```python
from build123d import *

# Parameters (mm, degrees)
F2_DEPTH      = 300
F3_W          = 8
F3_H          = 46
F4_DEPTH      = 5
F5_W          = 8
F5_H          = 46
F6_DEPTH      = 5
F7_W          = 50
F7_H          = 6
F8_DEPTH      = 5
F9_W          = 66
F9_H          = 45
F10_DEPTH     = 65.001
F11_R         = 2
F12_DEPTH     = 50.001
F13_T1_DEPTH  = 30
F13_T6_DEPTH  = 325
F13_T11_DEPTH = 325
F13_T16_DEPTH = 325
F13_T22_DEPTH = 325
F13_T27_DEPTH = 325
F13_T32_DEPTH = 325
F13_T37_DEPTH = 325
F13_T43_DEPTH = 325


# Not quite as in the source:
# - a fillet or chamfer that OpenCascade refuses, or shapes differently, is made with other operations: its cross-section is extruded or revolved along the edge and cut away or added


with BuildPart() as f2:
    # F1 (on face) → F2 (new body)
    with BuildSketch(Plane.XZ):
        Polygon((0, 0), (5, 0), (5, 45), (55, 45), (55, 0), (60, 0), (60, 50), (0, 50), align=None)
    extrude(amount=F2_DEPTH)

    # F3 (on face) → F4 (join)
    with BuildSketch(Plane.YZ.offset(60)):
        with Locations((-225, 25)):
            Rectangle(F3_W, F3_H)
        with Locations((-75, 25)):
            Rectangle(F3_W, F3_H)
    extrude(amount=F4_DEPTH)

    # F5 (on face) → F6 (join)
    with BuildSketch(Plane(origin=(0, 0, 0), x_dir=(0, -1, 0), z_dir=(-1, 0, 0))):
        with Locations((75, 25)):
            Rectangle(F5_W, F5_H)
        with Locations((225, 25)):
            Rectangle(F5_W, F5_H)
    extrude(amount=F6_DEPTH)

    # F7 (on face) → F8 (join)
    with BuildSketch(Plane(origin=(0, 0, 0), x_dir=(1, 0, 0), z_dir=(0, 0, -1))):
        with Locations((30, 74)):
            Rectangle(F7_W, F7_H)
        with Locations((30, 224)):
            Rectangle(F7_W, F7_H)
    extrude(amount=-F8_DEPTH)

    # F9 (on face) → F10 (cut, through all)
    with BuildSketch(Plane(origin=(0, 0, 0), x_dir=(0, -1, 0), z_dir=(-1, 0, 0))):
        Polygon((221, 45), (79, 45), (79, 2), (79, 0), (221, 0), (221, 2), align=None)
        with Locations((33, 22.5)):
            Rectangle(F9_W, F9_H)
        with Locations((267, 22.5)):
            Rectangle(F9_W, F9_H)
    extrude(amount=-F10_DEPTH, mode=Mode.SUBTRACT)

    # F11 (on Top) → F12 (cut, through all)
    with BuildSketch(Plane.XY):
        with Locations((-2.5, -75)):
            Circle(F11_R)
        with Locations((62.5, -75)):
            Circle(F11_R)
        with Locations((-2.5, -225)):
            Circle(F11_R)
        with Locations((62.5, -225)):
            Circle(F11_R)
    extrude(amount=F12_DEPTH, mode=Mode.SUBTRACT)

    # F13: fillet of radius 5 on 6 edges, made by hand

    # F13_s2 → F13_t1 (cut)
    with BuildSketch(Plane.XY.offset(32.5)):
        with BuildLine():
            ThreePointArc((0, -295), (1.4644660941, -298.5355339059), (5, -300))
            Line((5, -300), (0, -300))
            Line((0, -300), (0, -295))
        make_face()
        with BuildLine():
            ThreePointArc((60, -295), (58.5355339059, -298.5355339059), (55, -300))
            Line((55, -300), (60, -300))
            Line((60, -300), (60, -295))
        make_face()
        with BuildLine():
            ThreePointArc((60, -5), (58.5355339059, -1.4644660941), (55, 0))
            Line((55, 0), (60, 0))
            Line((60, 0), (60, -5))
        make_face()
        with BuildLine():
            ThreePointArc((0, -5), (1.4644660941, -1.4644660941), (5, 0))
            Line((5, 0), (0, 0))
            Line((0, 0), (0, -5))
        make_face()
    extrude(amount=F13_T1_DEPTH, mode=Mode.SUBTRACT)


with BuildPart() as f13_tool4:
    # F13_s5 → F13_t6 (new body)
    with BuildSketch(Plane.XZ.offset(-12.5)):
        with BuildLine():
            ThreePointArc((0, 45), (1.4644660941, 48.5355339059), (5, 50))
            Line((5, 50), (0, 50))
            Line((0, 50), (0, 45))
        make_face()
    extrude(amount=F13_T6_DEPTH)

    split(bisect_by=Plane.XZ.offset(71), keep=Keep.BOTTOM)


with BuildPart() as f2_1:
    add(f2.part)

    # F13_t3: cut F13_tool4
    add(f13_tool4.part, mode=Mode.SUBTRACT)


with BuildPart() as f13_tool9:
    # F13_s10 → F13_t11 (new body)
    with BuildSketch(Plane.XZ.offset(-12.5)):
        with BuildLine():
            ThreePointArc((0, 45), (1.4644660941, 48.5355339059), (5, 50))
            Line((5, 50), (0, 50))
            Line((0, 50), (0, 45))
        make_face()
    extrude(amount=F13_T11_DEPTH)

    split(bisect_by=Plane.XY.offset(48), keep=Keep.TOP)


with BuildPart() as f2_2:
    add(f2_1.part)

    # F13_t8: cut F13_tool9
    add(f13_tool9.part, mode=Mode.SUBTRACT)


with BuildPart() as f13_tool14:
    # F13_s15 → F13_t16 (new body)
    with BuildSketch(Plane.XZ.offset(-12.5)):
        with BuildLine():
            ThreePointArc((0, 45), (1.4644660941, 48.5355339059), (5, 50))
            Line((5, 50), (0, 50))
            Line((0, 50), (0, 45))
        make_face()
    extrude(amount=F13_T16_DEPTH)

    split(bisect_by=Plane.XZ.offset(79), keep=Keep.TOP)

    split(bisect_by=Plane.XZ.offset(221), keep=Keep.BOTTOM)


with BuildPart() as f2_3:
    add(f2_2.part)

    # F13_t13: cut F13_tool14
    add(f13_tool14.part, mode=Mode.SUBTRACT)


with BuildPart() as f13_tool20:
    # F13_s21 → F13_t22 (new body)
    with BuildSketch(Plane.XZ.offset(-12.5)):
        with BuildLine():
            ThreePointArc((0, 45), (1.4644660941, 48.5355339059), (5, 50))
            Line((5, 50), (0, 50))
            Line((0, 50), (0, 45))
        make_face()
    extrude(amount=F13_T22_DEPTH)

    split(bisect_by=Plane.XZ.offset(229), keep=Keep.TOP)


with BuildPart() as f2_4:
    add(f2_3.part)

    # F13_t19: cut F13_tool20
    add(f13_tool20.part, mode=Mode.SUBTRACT)


with BuildPart() as f13_tool25:
    # F13_s26 → F13_t27 (new body)
    with BuildSketch(Plane.XZ.offset(-12.5)):
        with BuildLine():
            ThreePointArc((60, 45), (58.5355339059, 48.5355339059), (55, 50))
            Line((55, 50), (60, 50))
            Line((60, 50), (60, 45))
        make_face()
    extrude(amount=F13_T27_DEPTH)

    split(bisect_by=Plane.XZ.offset(71), keep=Keep.BOTTOM)


with BuildPart() as f2_5:
    add(f2_4.part)

    # F13_t24: cut F13_tool25
    add(f13_tool25.part, mode=Mode.SUBTRACT)


with BuildPart() as f13_tool30:
    # F13_s31 → F13_t32 (new body)
    with BuildSketch(Plane.XZ.offset(-12.5)):
        with BuildLine():
            ThreePointArc((60, 45), (58.5355339059, 48.5355339059), (55, 50))
            Line((55, 50), (60, 50))
            Line((60, 50), (60, 45))
        make_face()
    extrude(amount=F13_T32_DEPTH)

    split(bisect_by=Plane.XY.offset(48), keep=Keep.TOP)


with BuildPart() as f2_6:
    add(f2_5.part)

    # F13_t29: cut F13_tool30
    add(f13_tool30.part, mode=Mode.SUBTRACT)


with BuildPart() as f13_tool35:
    # F13_s36 → F13_t37 (new body)
    with BuildSketch(Plane.XZ.offset(-12.5)):
        with BuildLine():
            ThreePointArc((60, 45), (58.5355339059, 48.5355339059), (55, 50))
            Line((55, 50), (60, 50))
            Line((60, 50), (60, 45))
        make_face()
    extrude(amount=F13_T37_DEPTH)

    split(bisect_by=Plane.XZ.offset(79), keep=Keep.TOP)

    split(bisect_by=Plane.XZ.offset(221), keep=Keep.BOTTOM)


with BuildPart() as f2_7:
    add(f2_6.part)

    # F13_t34: cut F13_tool35
    add(f13_tool35.part, mode=Mode.SUBTRACT)


with BuildPart() as f13_tool41:
    # F13_s42 → F13_t43 (new body)
    with BuildSketch(Plane.XZ.offset(-12.5)):
        with BuildLine():
            ThreePointArc((60, 45), (58.5355339059, 48.5355339059), (55, 50))
            Line((55, 50), (60, 50))
            Line((60, 50), (60, 45))
        make_face()
    extrude(amount=F13_T43_DEPTH)

    split(bisect_by=Plane.XZ.offset(229), keep=Keep.TOP)


with BuildPart() as f2_8:
    add(f2_7.part)

    # F13_t40: cut F13_tool41
    add(f13_tool41.part, mode=Mode.SUBTRACT)


solid = f2_8.part
```
Model file for the job. Use its own axes, mm. A direction names the side the tool comes from. Round coordinates to 2 decimals unless told otherwise and drop trailing zeros. Order: outer loops, then holes, each group sorted by start corner. A loop starts at its lowest first (then second) coordinate and runs counter-clockwise, first axis right, second up. Notation, with made-up numbers: (23.5, 86.25) -> (81.5, 86.25) arc R22 cw to (81.5, 116.25) -> close; hole circle Ø8 at (-9, 77). An arc over 180 degrees is marked (long way). Use one line per item in the form item = value.
Item 1: Flat gauge pins, fed straight in: pin 1 Ø1.5 at (x, y) = (-2, -227) entering from -Z; pin 2 Ø5 at (y, z) = (-203.5, 40.5) entering from +X; pin 3 Ø3 at (x, y) = (50.5, -88) entering from -Z; pin 4 Ø1.5 at (x, y) = (58, -257.5) entering from +Z. Where does each tip first touch, or does it go through?
Returned:
pin_1 = 2
pin_2 = through
pin_3 = 45
pin_4 = 49.47
Item 2: Cut at B-B, the plane x = 16. Write the cut outline in (y, z).
Returned:
outline = (-300, 45) -> (0, 45) -> (0, 50) -> (-300, 50) -> close; (-227, 0) -> (-221, 0) -> (-221, 5) -> (-227, 5) -> close; (-77, 0) -> (-71, 0) -> (-71, 5) -> (-77, 5) -> close
Item 3: Tool access for faces 1 (the face through (2, -234, 22)), 2 (the face through (-1, -227, 2)), 3 (the face through (30, -74, 5)), 4 (the face through (2, -66, 22)), 5 (the face through (30, -71, 2)): list every direction of +Z, -Z, +X, -X, +Y, -Y with a clear straight run to the whole face (end or side of a thin tool).
Returned:
face_1 = -Z, +X, -X, -Y
face_2 = -Z, -X, +Y, -Y
face_3 = +Y, -Y
face_4 = -Z, +X, -X, +Y
face_5 = -Z, +Y
Item 4: Cut at A-A, the plane z = 30. Write the cut outline in (x, y).
Returned:
outline = (-5, -229) -> (0, -229) -> (0, -234) -> (5, -234) -> (5, -221) -> (-5, -221) -> close; (-5, -79) -> (5, -79) -> (5, -66) -> (0, -66) -> (0, -71) -> (-5, -71) -> close; (55, -234) -> (60, -234) -> (60, -229) -> (65, -229) -> (65, -221) -> (55, -221) -> close; (55, -79) -> (65, -79) -> (65, -71) -> (60, -71) -> (60, -66) -> (55, -66) -> close; hole circle Ø4 at (-2.5, -225); hole circle Ø4 at (-2.5, -75); hole circle Ø4 at (62.5, -225); hole circle Ø4 at (62.5, -75)
Item 5: Pull direction Y, two halves, no side cores. Call faces 6 (the face through (-3, -71, 25)), 7 (the face through (65, -225, 25)), 8 (the face through (60, -79, 24)): released by +Y, released by -Y, zero draft, split by the parting line, or undercut.
Returned:
face_6 = released by +Y
face_7 = zero draft
face_8 = undercut
Item 6: Drill centre lines: line 1 (X direction, y = -225, z = 23); line 2 (Y direction, x = 62.5, z = 37.5); line 3 (Y direction, x = -2, z = 20). Where is each one in solid material? Low to high.
Returned:
line_1 = -5 to -4.5, -0.5 to 5, 55 to 60.5, 64.5 to 65
line_2 = -229 to -227, -223 to -221, -79 to -77, -73 to -71
line_3 = -229 to -226.94, -223.06 to -221, -79 to -76.94, -73.06 to -71
Item 7: Cut at C-C, the plane y = -184.5. Write the cut outline in (x, z), and give its area (3 significant figures).
Returned:
outline = (0, 45) -> (60, 45) arc R5 ccw to (55, 50) -> (5, 50) arc R5 ccw to start
area = 289 mm^2
